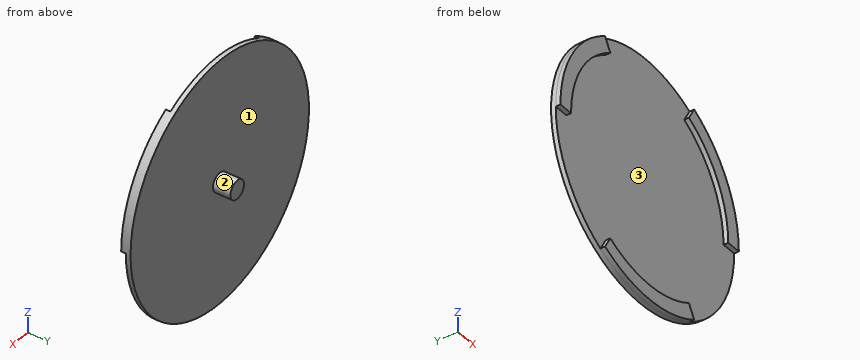
```python
from build123d import *

# Parameters (mm, degrees)
SKETCH1_W           = 105
SKETCH1_H           = 8
CUT_EXTRUDE1_DEPTH  = 4
BOSS_EXTRUDE1_DEPTH = 4
BOSS_EXTRUDE2_DEPTH = 4
SKETCH5_W           = 8
SKETCH5_H           = 15


with BuildPart() as part:
    # Sketch1 → Revolve1 (revolve)
    with BuildSketch(Plane.XY):
        with Locations((52.5, 4)):
            Rectangle(SKETCH1_W, SKETCH1_H)
    revolve(axis=Axis((0, 8, 0), (0, -1, 0)))

    # Sketch2 → Cut-Extrude1 (cut)
    with BuildSketch(Plane.XZ):
        with BuildLine():
            Line((46.25, 80.10734985), (52.5, 90.932667397))
            ThreePointArc((52.5, 90.932667397), (-90.932667397, -52.5), (105, 0))
            Line((105, 0), (92.5, 0))
            ThreePointArc((92.5, 0), (80.10734985, 46.25), (46.25, 80.10734985))
        make_face()
    extrude(amount=-CUT_EXTRUDE1_DEPTH, mode=Mode.SUBTRACT)

    # Sketch3 → Boss-Extrude1 (add)
    with BuildSketch(Plane.XZ.offset(-4)):
        with BuildLine():
            Line((-92.5, 0), (-105, 0))
            ThreePointArc((-105, 0), (-90.932667397, 52.5), (-52.5, 90.932667397))
            Line((-52.5, 90.932667397), (-46.25, 80.10734985))
            ThreePointArc((-46.25, 80.10734985), (-80.10734985, 46.25), (-92.5, 0))
        make_face()
    extrude(amount=BOSS_EXTRUDE1_DEPTH)

    # Sketch4 → Boss-Extrude2 (add)
    with BuildSketch(Plane.XZ.offset(-4)):
        with BuildLine():
            Line((-52.5, -90.932667397), (-46.25, -80.10734985))
            ThreePointArc((-46.25, -80.10734985), (0, -92.5), (46.25, -80.10734985))
            Line((46.25, -80.10734985), (52.5, -90.932667397))
            ThreePointArc((52.5, -90.932667397), (0, -105), (-52.5, -90.932667397))
        make_face()
    extrude(amount=BOSS_EXTRUDE2_DEPTH)

    # Sketch5 → Revolve2 (revolve)
    with BuildSketch(Plane.XY):
        with Locations((4, 15.5)):
            Rectangle(SKETCH5_W, SKETCH5_H)
    revolve(axis=Axis((0, 23, 0), (0, -1, 0)))


solid = part.part
```
For this review, take the finished solid that the model builds, in its own axes (mm). Face numbers are marked on the shaded views. Round coordinates to 2 decimals unless told otherwise and drop trailing zeros. Write each loop counter-clockwise with the first axis right and the second up, starting at its lowest first coordinate (ties: lowest second). Pieces come first, ordered by that corner, then holes.
1) Mouldability with a two-part tool opening along X and no side actions: class the marked faces 1, 2 and 3 as +X half, -X half, draft (parallel to the pull), parting line (faces both ways), or undercut.
Answer below:
face 1: draft
face 2: parting line
face 3: undercut
2) Insertion check: pin 1 Ø1.5 at (x, z) = (-11.5, -34) entering from +Y; pin 2 Ø2 at (x, z) = (62, 3.5) entering from -Y; pin 3 Ø3 at (x, y) = (-96, 1) entering from -Z. Each pin has a flat end and moves straight along its axis. Give the tip position at first contact, or say it passes through.
Answer below:
pin 1: stops at y = 8
pin 2: stops at y = 4
pin 3: stops at z = 0
3) Take a section at C-C on z = -52.5. Give the boundary of the cut face in (x, y).
Answer below:
outline: (-90.93, 4) - (90.93, 4) - (90.93, 8) - (-90.93, 8) - close
4) For line 1 along Y through (x, z) = (63.5, 58); line 2 along Y through (x, z) = (-94.5, 7); line 3 along Z through (x, y) = (23, 6.25), list the stretches that pass through material, from the lowest coordinate up.
Answer below:
line 1: y = 4 to 8
line 2: y = 0 to 8
line 3: z = -102.45 to 102.45
5) Take a section at A-A on x = 0. Give the boundary of the cut face in (y, z).
Answer below:
outline: (0, -105) - (8, -105) - (8, -8) - (23, -8) - (23, 8) - (8, 8) - (8, 105) - (4, 105) - (4, -92.5) - (0, -92.5) - close
6) Take a section at D-D on x = 23.5. Give the boundary of the cut face in (y, z).
Answer below:
outline: (0, -102.34) - (8, -102.34) - (8, 102.34) - (4, 102.34) - (4, -89.47) - (0, -89.47) - close
7) Take a section at B-B on y = 14. Give the boundary of the cut face in (x, z).
Answer below:
outline: circle Ø16 at (0, 0)
